For this review, take the finished solid that the model builds, in its own axes (mm). A direction names the side the tool comes from. Coordinates: 2 decimals unless noted, no trailing zeros. Loops run counter-clockwise (first coordinate to the right, second up) from the corner with the lowest first, then second, coordinate; pieces in that order, holes last. Notation, with made-up numbers: M -16.75,23.25 L -9.75,23.25 A23 ccw -9.75,56.25 Z; hole C 78,7 d5. An arc over 180 degrees is marked long. Put each result on its own line as item: value.
```python
from build123d import *

# Parameters (mm, degrees)
F0_R     = 7.5
F0_R_2   = 1.5
F1_DEPTH = 15
F2_SIZE  = 5
F3_R     = 4
F4_DEPTH = 2


with BuildPart() as f1:
    # F0 (on Top) → F1 (new body)
    with BuildSketch(Plane.XY):
        Circle(F0_R)
        Circle(F0_R_2, mode=Mode.SUBTRACT)
    extrude(amount=F1_DEPTH)

    # F2
    f2_edges = [f1.edges().sort_by_distance(p)[0] for p in [
        (-7.5, 0, 15),
    ]]
    chamfer(f2_edges, length=F2_SIZE)

    # F3 (on face) → F4 (cut)
    with BuildSketch(Plane(origin=(0, 0, 0), x_dir=(1, 0, 0), z_dir=(0, 0, -1))):
        Circle(F3_R)
    extrude(amount=-F4_DEPTH, mode=Mode.SUBTRACT)


solid = f1.part
```
(1) Tool access review of faces 1 (the cylindrical face through (-7.493, 0.33, 4.93)), 2 (the flat face through (2, 0, 2)): name each direction out of +Z, -Z, +X, -X, +Y, -Y from which nothing blocks a thin tool from reaching the whole face with its end or side.
Determined:
face 1: +Z, -Z
face 2: -Z
(2) Wall thickness on line 1 along Y through (x, z) = (0, 6); line 2 along Y through (x, z) = (0, 1.15); line 3 along Z through (x, y) = (-2, 1): over which ranges is each line inside the solid? List them lowest first. Write a range as [from, to].
Determined:
line 1: y = [-7.5, -1.5], [1.5, 7.5]
line 2: y = [-7.5, -4], [4, 7.5]
line 3: z = [2, 15]
(3) Add section C-C (z = 4.5). Write out the cut boundary in (x, y).
Determined:
outline: C 0,0 d15; hole C 0,0 d3
(4) Draft analysis for pull direction X (two halves, no side actions). For faces 3 (the flat face through (2, 0, 15)), 4 (the cylindrical face through (-1.5, 0.07, 8.41)), 5 (the conical face through (-0.595, -2.678, 14.757)), state which applies: +X half, -X half, draft (parallel to the pull), parting line (faces both ways), or undercut.
Determined:
face 3: draft
face 4: undercut
face 5: parting line
(5) Add section A-A (x = 0). Write out the cut boundary in (y, z).
Determined:
outline: M -7.5,0 L -4,0 L -4,2 L -1.5,2 L -1.5,15 L -2.5,15 L -7.5,10 Z; M 1.5,2 L 4,2 L 4,0 L 7.5,0 L 7.5,10 L 2.5,15 L 1.5,15 Z
(6) Add section D-D (z = 12). Write out the cut boundary in (x, y), plus the area to 3 significant figures.
Determined:
outline: C 0,0 d11; hole C 0,0 d3
area: 88.0 mm^2
(7) For pin 1 (1.5 mm diameter, centred on x = -2, z = 7, fed in from -Y); pin 2 (3 mm diameter, centred on x = -4, z = 8, fed in from -Y); pin 3 (1 mm diameter, centred on y = -5.5, z = 4.5, fed in from +X), all flat-tipped, find the tip position at first contact; note any pin that passes through.
Determined:
pin 1: stops at y = -7.4
pin 2: stops at y = -7.07
pin 3: stops at x = 5.59
